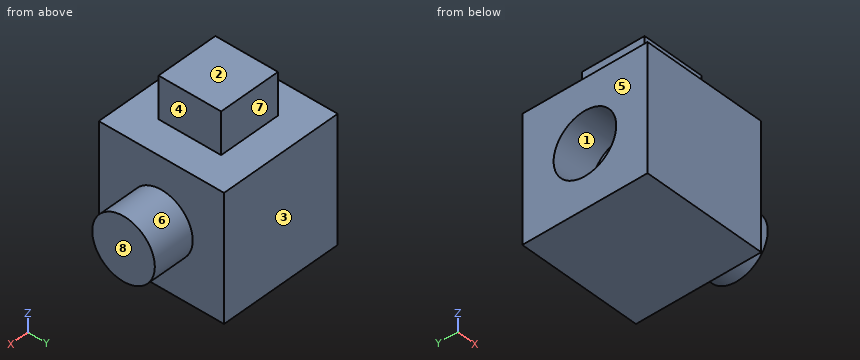
from build123d import *

# Parameters (mm, degrees)
F0_W     = 76.2
F0_H     = 76.2
F1_DEPTH = 76.2
F2_W     = 38.1
F2_H     = 38.1
F5_DEPTH = 25.4
F3_R     = 19.05
F6_DEPTH = 25.4
F4_R     = 19.05
F7_DEPTH = 25.4


with BuildPart() as f1:
    # F0 (on Top) → F1 (new body)
    with BuildSketch(Plane.XY):
        with Locations((-29.714826, -11.961539)):
            Rectangle(F0_W, F0_H)
    extrude(amount=F1_DEPTH)

    # F2 (on face) → F5 (join)
    with BuildSketch(Plane.XY.offset(76.2)):
        with Locations((-29.714826, -11.961539)):
            Rectangle(F2_W, F2_H)
    extrude(amount=F5_DEPTH)

    # F3 (on face) → F6 (join)
    with BuildSketch(Plane.YZ.offset(8.385174)):
        with Locations((-11.961539, 38.1)):
            Circle(F3_R)
    extrude(amount=F6_DEPTH)

    # F4 (on face) → F7 (cut)
    with BuildSketch(Plane(origin=(-67.814826, 0, 0), x_dir=(0, -1, 0), z_dir=(-1, 0, 0))):
        with Locations((11.961539, 38.1)):
            Circle(F4_R)
    extrude(amount=-F7_DEPTH, mode=Mode.SUBTRACT)


solid = f1.part
Verification items for the finished model (mm, model axes). Face numbers are marked on the shaded views. A direction names the side the tool comes from. Round coordinates to 2 decimals unless told otherwise and drop trailing zeros. Loops run counter-clockwise (first coordinate to the right, second up) from the corner with the lowest first, then second, coordinate; pieces in that order, holes last. Notation, with made-up numbers: (5, 14.25) - (17, 14.25) arc R9 ccw to (17, 21.25) - close; hole circle Ø5 at (12, -19). An arc over 180 degrees is marked (long way). Use one line per item in the form item = value.
1. Section check D-D on y = 18. Record the cut outline in (x, z).
A:
outline = (-67.81, 0) - (8.39, 0) - (8.39, 76.2) - (-67.81, 76.2) - close
2. Access from +Z, -Z, +X, -X, +Y, -Y to the whole of each face (thin tool, end or side, straight path). Record for the marked faces 4, 5, 6, 7 and 8.
A:
face_4 = +Z, +X, +Y, -Y
face_5 = +Z, -Z, -X, +Y, -Y
face_6 = +X
face_7 = +Z, +X, -X, +Y
face_8 = +Z, -Z, +X, +Y, -Y
3. Scan lines: probe 1 along Y at (x, z) = (-51, 38); probe 2 along X at (y, z) = (12.5, 19.5); probe 3 along X at (y, z) = (-4, 45.5). Record each from-to range of solid material in increasing order.
A:
probe_1 = -50.06 to -31.01, 7.09 to 26.14
probe_2 = -67.81 to 8.39
probe_3 = -42.41 to 33.79
4. Gauge pin test, flat ends, axial feed: pin 1 Ø12 at (x, y) = (19, -1) entering from -Z; pin 2 Ø20.5 at (y, z) = (-5, 94) entering from +X; pin 3 Ø4 at (x, y) = (-53.5, 5.5) entering from +Z. Record the tip position at first contact, or that the pin passes through.
A:
pin_1 = 19.71
pin_2 = -10.66
pin_3 = 76.2
5. Section check A-A on z = 38.1. Record the cut outline in (x, y), and give its area (3 significant figures).
A:
outline = (-67.81, -50.06) - (8.39, -50.06) - (8.39, -31.01) - (33.79, -31.01) - (33.79, 7.09) - (8.39, 7.09) - (8.39, 26.14) - (-67.81, 26.14) - (-67.81, 7.09) - (-42.41, 7.09) - (-42.41, -31.01) - (-67.81, -31.01) - close
area = 5,810 mm²
6. Section check C-C on y = -5.5. Record the cut outline in (x, z), and give its area (3 significant figures).
A:
outline = (-67.81, 0) - (8.39, 0) - (8.39, 20.18) - (33.79, 20.18) - (33.79, 56.02) - (8.39, 56.02) - (8.39, 76.2) - (-10.66, 76.2) - (-10.66, 101.6) - (-48.76, 101.6) - (-48.76, 76.2) - (-67.81, 76.2) - (-67.81, 56.02) - (-42.41, 56.02) - (-42.41, 20.18) - (-67.81, 20.18) - close
area = 6,770 mm²
7. Draft check along Z on the marked faces 1, 2 and 3. Enter one of: pulls with the +Z half, pulls with the -Z half, needs draft (parallel to the pull), parting line crosses it, or undercut.
A:
face_1 = undercut
face_2 = pulls with the +Z half
face_3 = needs draft
8. Section check B-B on x = -13. Record the cut outline in (y, z), and give its area (3 significant figures).
A:
outline = (-50.06, 0) - (26.14, 0) - (26.14, 76.2) - (7.09, 76.2) - (7.09, 101.6) - (-31.01, 101.6) - (-31.01, 76.2) - (-50.06, 76.2) - close
area = 6,770 mm²
